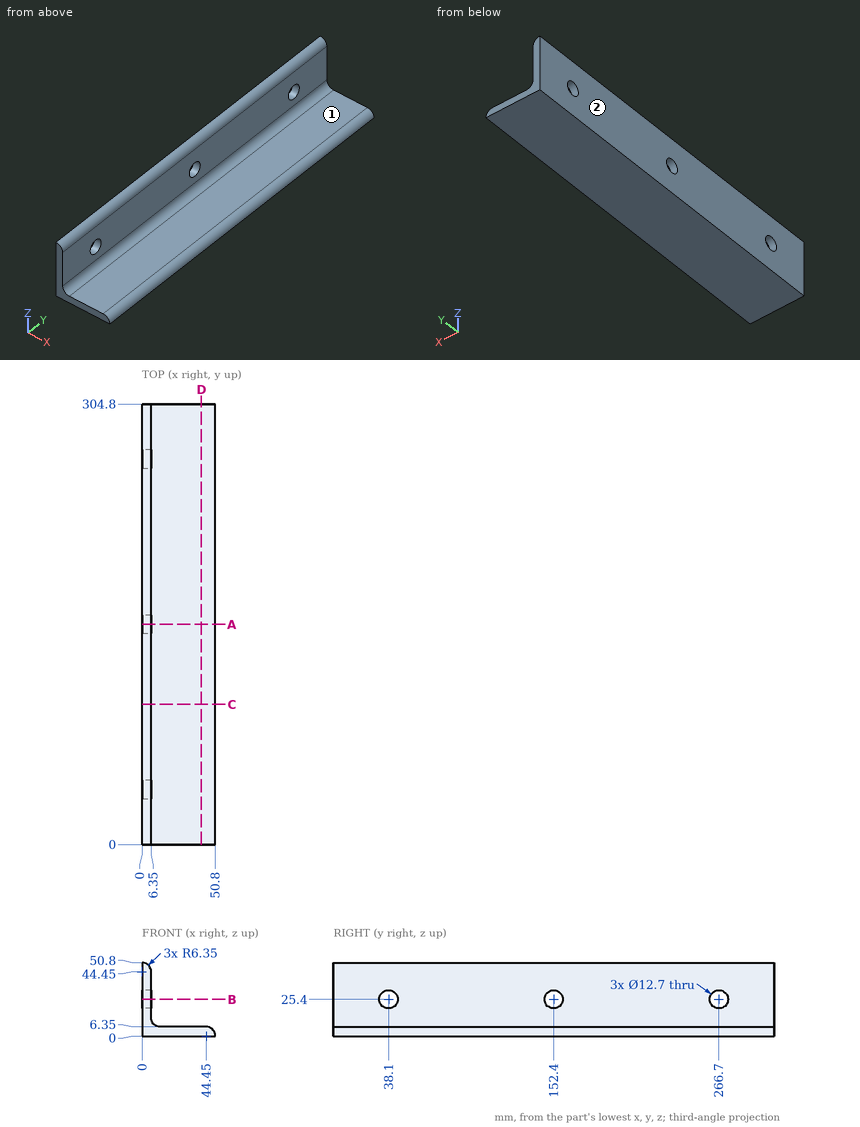
Verification items for this drawing (mm, ordinates from the low corner). A direction names the side the tool comes from. Round coordinates to 2 decimals unless told otherwise and drop trailing zeros. Write each loop counter-clockwise with the first axis right and the second up, starting at its lowest first coordinate (ties: lowest second). Pieces come first, ordered by that corner, then holes. Notation, with made-up numbers: M 80,-39 L 131,-39 A14 ccw 131,-25 Z; hole C 15,35 d1. An arc over 180 degrees is marked long. Write item = value, one per line. Start each with the question number.
1. Section check D-D, the plane x = 41. Record the cut outline in (y, z).
2. Section check A-A, the plane y = 152.4. Record the cut outline in (x, z).
3. Tool access check on the marked faces 1 and 2. Record the directions out of +Z, -Z, +X, -X, +Y, -Y that give a thin tool (end or side, any length) a straight path to the whole face; none if there is none.
4. Scan lines: line 1 (Y direction, x = 4, z = 25); line 2 (X direction, y = 268, z = 34). Record each from-to range of solid material in increasing order. Write a range as [from, to].
5. Gauge pin test, flat ends, axial feed: pin 1 (3 mm diameter, centred on y = 44, z = 15.5, fed in from +X); pin 2 (11.5 mm diameter, centred on y = 38.1, z = 25.4, fed in from -X); pin 3 (8 mm diameter, centred on y = 148.5, z = 7.5, fed in from +X). Record the tip position at first contact, or that the pin passes through.
6. Section check C-C, the plane y = 97. Record the cut outline in (x, z), then the cut area to 3 significant figures.
7. Section check B-B, the plane z = 25.4. Record the cut outline in (x, y), then the cut area to 3 significant figures.
Results found:
q1.outline = M 0,0 L 304.8,0 L 304.8,6.35 L 0,6.35 Z
q2.outline = M 0,0 L 50.8,0 A6.35 ccw 44.45,6.35 L 12.7,6.35 A6.35 cw 6.35,12.7 L 6.35,19.05 L 0,19.05 Z; M 0,31.75 L 6.35,31.75 L 6.35,44.45 A6.35 ccw 0,50.8 Z
q3.face_1 = +Z, +X, +Y, -Y
q3.face_2 = +Z, -Z, -X, +Y, -Y
q4.line_1 = [0, 31.76], [44.44, 146.06], [158.74, 260.36], [273.04, 304.8]
q4.line_2 = [0, 6.35]
q5.pin_1 = 6.35
q5.pin_2 = through
q5.pin_3 = 49.75
q6.outline = M 0,0 L 50.8,0 A6.35 ccw 44.45,6.35 L 12.7,6.35 A6.35 cw 6.35,12.7 L 6.35,44.45 A6.35 ccw 0,50.8 Z
q6.area = 596 mm^2
q7.outline = M 0,0 L 6.35,0 L 6.35,31.75 L 0,31.75 Z; M 0,44.45 L 6.35,44.45 L 6.35,146.05 L 0,146.05 Z; M 0,158.75 L 6.35,158.75 L 6.35,260.35 L 0,260.35 Z; M 0,273.05 L 6.35,273.05 L 6.35,304.8 L 0,304.8 Z
q7.area = 1,690 mm^2
